```python
from build123d import *

# Parameters (mm, degrees)
SKETCH1_R           = 2.0193
BOSS_EXTRUDE1_DEPTH = 165.1


with BuildPart() as part:
    # Sketch1 → Boss-Extrude1 (new body)
    with BuildSketch(Plane.XY):
        with BuildLine():
            ThreePointArc((-2.623741315, 6.35), (-3.43535, 5.950200742), (-4.187390656, 5.447226632))
            Line((-4.187390656, 5.447226632), (-6.811131972, 0.902773368))
            ThreePointArc((-6.811131972, 0.902773368), (-6.8707, 0), (-6.811131972, -0.902773368))
            Line((-6.811131972, -0.902773368), (-4.187390656, -5.447226632))
            ThreePointArc((-4.187390656, -5.447226632), (-3.43535, -5.950200742), (-2.623741315, -6.35))
            Line((-2.623741315, -6.35), (2.623741315, -6.35))
            ThreePointArc((2.623741315, -6.35), (3.43535, -5.950200742), (4.187390656, -5.447226632))
            Line((4.187390656, -5.447226632), (6.811131972, -0.902773368))
            ThreePointArc((6.811131972, -0.902773368), (6.8707, 0), (6.811131972, 0.902773368))
            Line((6.811131972, 0.902773368), (4.187390656, 5.447226632))
            ThreePointArc((4.187390656, 5.447226632), (3.43535, 5.950200742), (2.623741315, 6.35))
            Line((2.623741315, 6.35), (-2.623741315, 6.35))
        make_face()
        Circle(SKETCH1_R, mode=Mode.SUBTRACT)
    extrude(amount=BOSS_EXTRUDE1_DEPTH)


solid = part.part
```
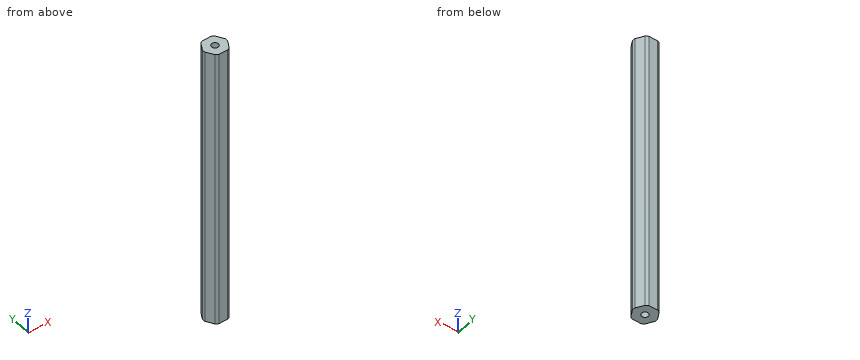
The listing builds one solid part. Answer for the finished solid, in the listing's coordinates (mm). Coordinates: 2 decimals unless noted, no trailing zeros. Write each loop counter-clockwise with the first axis right and the second up, starting at its lowest first coordinate (ties: lowest second). Pieces come first, ordered by that corner, then holes. Notation, with made-up numbers: (8.25, 21) -> (67.25, 21) arc R34 ccw to (67.25, 60) -> close; hole circle Ø10 at (19, 76.25). An arc over 180 degrees is marked (long way). Write each question's results on one line, items separated by ' | '. Start each with the question number.
1) Flat-ended cylindrical pins translate along their axes: pin 1 Ø3 at (x, z) = (-5, 81) entering from -Y; pin 2 Ø4 at (y, z) = (3, 83) entering from -X (3 decimals); pin 3 Ø1.5 at (y, z) = (-2, 119.5) entering from -X; pin 4 Ø2 at (x, z) = (-3, 82.5) entering from +Y. Find the tip coordinate at first contact, or state that the pin passes through.
2) A cutting plane is placed at A-A (z = 18.5). Determine the outline of the cut face in (x, y).
3) A cutting plane is placed at B-B (x = 0). Determine the outline of the cut face in (y, z).
4) Straight lines are drawn through the part: probe 1 along Y at (x, z) = (0, 74.5); probe 2 along Y at (x, z) = (1, 74); probe 3 along X at (y, z) = (-0.5, 22). For each, find the intervals that lie inside material, in ascending order.
5) A cutting plane is placed at C-C (y = -4). Determine the outline of the cut face in (x, z), then the cut area to 3 significant figures.
Values follow:
1) pin 1: y = -5.91 | pin 2: x = -6.755 | pin 3: x = -6.61 | pin 4: y = 6.35
2) outline: (-6.81, -0.9) -> (-4.19, -5.45) arc R6.87 ccw to (-2.62, -6.35) -> (2.62, -6.35) arc R6.87 ccw to (4.19, -5.45) -> (6.81, -0.9) arc R6.87 ccw to (6.81, 0.9) -> (4.19, 5.45) arc R6.87 ccw to (2.62, 6.35) -> (-2.62, 6.35) arc R6.87 ccw to (-4.19, 5.45) -> (-6.81, 0.9) arc R6.87 ccw to start; hole circle Ø4.04 at (0, 0)
3) outline: (-6.35, 0) -> (-2.02, 0) -> (-2.02, 165.1) -> (-6.35, 165.1) -> close; (2.02, 0) -> (6.35, 0) -> (6.35, 165.1) -> (2.02, 165.1) -> close
4) probe 1: -6.35 to -2.02, 2.02 to 6.35 | probe 2: -6.35 to -1.75, 1.75 to 6.35 | probe 3: -6.85 to -1.96, 1.96 to 6.85
5) outline: (-5.02, 0) -> (5.02, 0) -> (5.02, 165.1) -> (-5.02, 165.1) -> close | area: 1,660 mm²
